Verification items for this drawing (mm, ordinates from the low corner). A direction names the side the tool comes from. Give positions to 0.01 mm unless a question says otherwise; leave off trailing zeros. Loops run counter-clockwise (first coordinate to the right, second up) from the corner with the lowest first, then second, coordinate; pieces in that order, holes last. Notation, with made-up numbers: M 7.25,24.25 L 36.25,24.25 A13 cw 36.25,28.25 Z; hole C 22.5,43.25 d8. An arc over 180 degrees is marked long. Put each result on its own line as item: value. Start each with the question number.
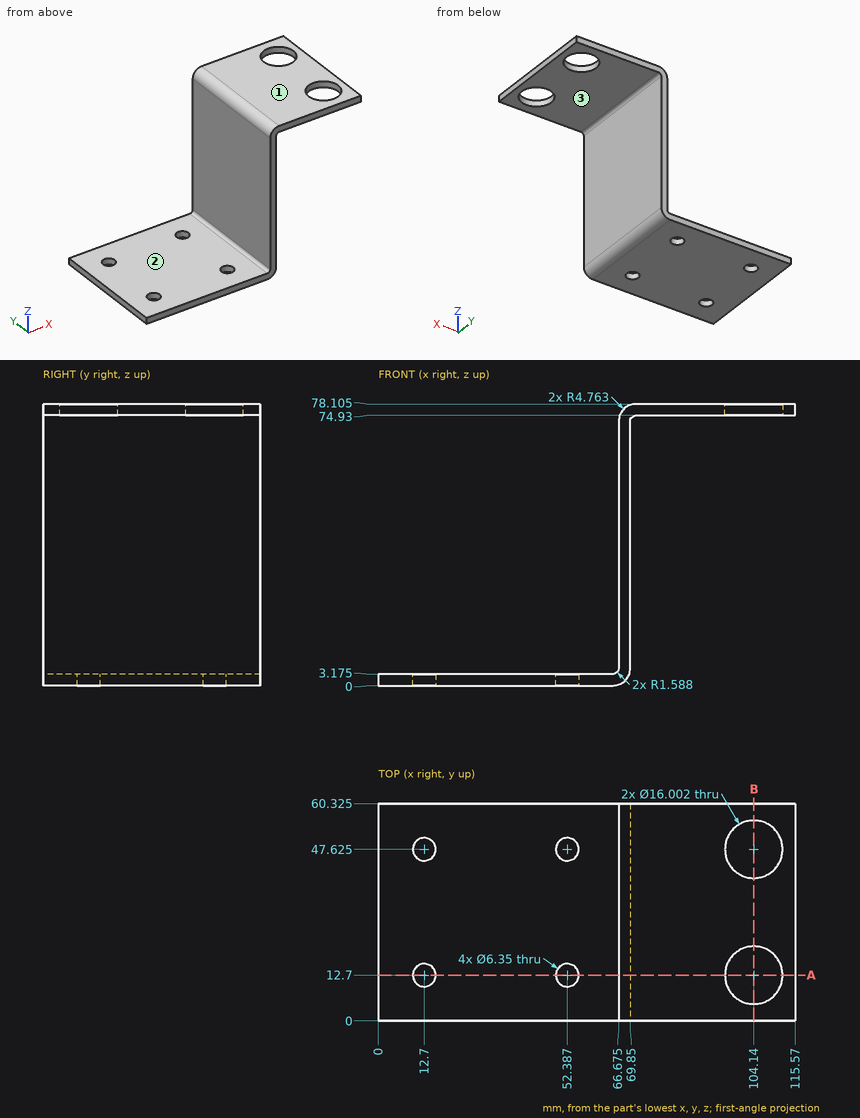
Q1. Cross-section at A-A, the plane y = 12.7. State how many separate pieces and enclosed holes the cut face has, then the cut area to 3 significant figures.
Q2. Scan lines: L1, parallel to Y at x = 104.14, z = 76.45 (1 decimal); L2, parallel to Z at x = 96, y = 32.5 (1 decimal); L3, parallel to X at y = 12, z = 1 (1 decimal). Record each from-to range of solid material in increasing order.
Q3. Cross-section at B-B, the plane x = 104.14. Record the boundary of the cut face in (y, z) (1 decimal).
Q4. Set-up check for the marked faces 1, 2 and 3: record each of +Z, -Z, +X, -X, +Y, -Y from which the full face is reachable in a straight line by a thin tool's end or side.
Q5. Go/stop test with flat-tipped pins: pin 1 (12 mm diameter, centred on y = 22.5, z = 69.5, fed in from -X) (1 decimal); pin 2 (1.5 mm diameter, centred on y = 22.5, z = 65, fed in from +X); pin 3 (10 mm diameter, centred on x = 94, y = 39.5, fed in from -Z). Record where each tip stops, or that it passes through.
Ans:
1. separate pieces: 4
1. enclosed holes: 0
1. area: 505 mm^2
2. L1: y = 0 to 4.7, 20.7 to 39.6, 55.6 to 60.3
2. L2: z = 74.9 to 78.1
2. L3: x = 0 to 9.6, 15.8 to 49.3, 55.5 to 68
3. outline: M 0,74.9 L 4.7,74.9 L 4.7,78.1 L 0,78.1 Z; M 20.7,74.9 L 39.6,74.9 L 39.6,78.1 L 20.7,78.1 Z; M 55.6,74.9 L 60.3,74.9 L 60.3,78.1 L 55.6,78.1 Z
4. face 1: +Z, +X, -X, +Y, -Y
4. face 2: +Z, -X, +Y, -Y
4. face 3: -Z, +X, +Y, -Y
5. pin 1: stops at x = 66.7
5. pin 2: stops at x = 69.85
5. pin 3: stops at z = 74.93
